Can you work these out from the model? Positions are in its coordinate system, mm. Face numbers are marked on the shaded views. Coordinates: 2 decimals unless noted, no trailing zeros. Loops run counter-clockwise (first coordinate to the right, second up) from the corner with the lowest first, then second, coordinate; pieces in that order, holes last. Notation, with made-up numbers: M -15.75,71.25 L 21.25,71.25 A24 ccw 21.25,102.25 Z; hole C 83.25,-14 d7. An arc over 180 degrees is marked long. Return JSON: item names as keys, results as strings. Group by question number.
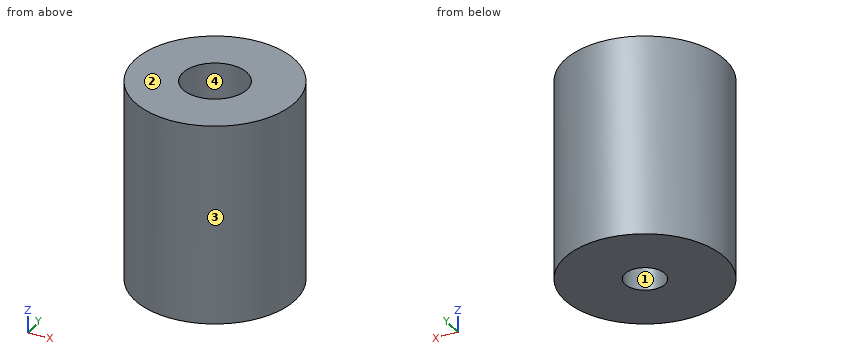
```python
from build123d import *

# Parameters (mm, degrees)
SKETCH_R        = 10
PAD_DEPTH       = 25
SKETCH001_R     = 4
POCKET_DEPTH    = 12.5
SKETCH002_R     = 2.5
POCKET001_DEPTH = 12.5


with BuildPart() as part:
    # Sketch → Pad (new body)
    with BuildSketch(Plane.XY):
        Circle(SKETCH_R)
    extrude(amount=PAD_DEPTH)

    # Sketch001 (on Face3 of Pad) → Pocket (cut)
    with BuildSketch(Plane.XY.offset(25)):
        Circle(SKETCH001_R)
    extrude(amount=-POCKET_DEPTH, mode=Mode.SUBTRACT)

    # Sketch002 (on Face2 of Pocket) → Pocket001 (cut)
    with BuildSketch(Plane(origin=(0, 0, 0), x_dir=(1, 0, 0), z_dir=(0, 0, -1))):
        Circle(SKETCH002_R)
    extrude(amount=-POCKET001_DEPTH, mode=Mode.SUBTRACT)


solid = part.part
```
1) If I drill on line 1 (Y direction, x = 0, z = 18.75); line 2 (Y direction, x = 0, z = 8); line 3 (Z direction, x = 3.5, y = 1.75), over which ranges is the centre line in solid material (lowest first)? Write a range as from..to.
2) For pin 1 (6 mm diameter, centred on x = 0, y = 0, fed in from +Z); pin 2 (10 mm diameter, centred on x = -5, z = 6, fed in from -Y); pin 3 (4 mm diameter, centred on y = 2.5, z = 13.5, fed in from -X); pin 4 (6 mm diameter, centred on y = 7, z = 19.5, fed in from +X), each with a flat end and sliding along its axis, tell me the tip position at first contact or that it passes through.
3) Suppose I cut it at C-C, the plane z = 22.75. List the corners of the cut face in (x, y) for me, then the cut area to 3 significant figures.
4) Suppose I cut it at D-D, the plane x = 3.25. List the corners of the cut face in (y, z) for me, then the cut area to 3 significant figures.
5) Suppose I cut it at A-A, the plane x = 0. List the corners of the cut face in (y, z) for me, then the cut area to 4 significant figures.
6) If we mould it in two halves opening along Y, with no side actions, what happens to the marked faces 1, 2, 3 and 4? For each: +Y half, -Y half, draft (parallel to the pull), parting line (faces both ways), or undercut.
Returned:
{
 "1": {"line 1": "y = -10..-4, 4..10", "line 2": "y = -10..-2.5, 2.5..10", "line 3": "z = 0..12.5"},
 "2": {"pin 1": "stops at z = 12.5", "pin 2": "stops at y = -10", "pin 3": "stops at x = -9.99", "pin 4": "stops at x = 9.17"},
 "3": {"outline": "C 0,0 d20; hole C 0,0 d8", "area": "264 mm²"},
 "4": {"outline": "M -9.46,0 L 9.46,0 L 9.46,25 L 2.33,25 L 2.33,12.5 L -2.33,12.5 L -2.33,25 L -9.46,25 Z", "area": "415 mm²"},
 "5": {"outline": "M -10,0 L -2.5,0 L -2.5,12.5 L -4,12.5 L -4,25 L -10,25 Z; M 2.5,0 L 10,0 L 10,25 L 4,25 L 4,12.5 L 2.5,12.5 Z", "area": "337.5 mm²"},
 "6": {"face 1": "undercut", "face 2": "draft", "face 3": "parting line", "face 4": "undercut"}
}
